Part model, mm, in its own coordinate system. Round coordinates to 2 decimals unless told otherwise and drop trailing zeros. Loops run counter-clockwise (first coordinate to the right, second up) from the corner with the lowest first, then second, coordinate; pieces in that order, holes last.
(1) Cut at B-B on z = 3. List the corners of the cut face in (x, y) (3 decimals), then the cut area to 3 significant figures.
(2) Cut at A-A on y = 60. List the corners of the cut face in (x, z) (3 decimals), then the cut area to 3 significant figures.
(3) Cut at C-C on x = 52. List the corners of the cut face in (y, z), then the cut area to 3 significant figures.
(4) Probe probe 1 along Z at (x, y) = (52, 53); probe 2 along X at (y, z) = (24, 2.4); probe 3 along X at (y, z) = (142, 4.1). List the from-to ranges inside material, lowest first.
from build123d import *

# Parameters (mm, degrees)
F0_W     = 94
F0_H     = 165.2
F1_DEPTH = 6
F2_R     = 2.5
F3_DEPTH = 165.201
F4_SIZE  = 2


with BuildPart() as f1:
    # F0 (on Top) → F1 (new body)
    with BuildSketch(Plane.XY):
        with Locations((47, 82.6)):
            Rectangle(F0_W, F0_H)
    extrude(amount=F1_DEPTH)

    # F2 (on face) → F3 (cut, through all)
    with BuildSketch(Plane.XZ):
        with Locations((42.305, 3)):
            Circle(F2_R)
        with Locations((51.695, 3)):
            Circle(F2_R)
    extrude(amount=-F3_DEPTH, mode=Mode.SUBTRACT)

    # F4
    f4_edges = [f1.edges().sort_by_distance(p)[0] for p in [
        (0, 82.6, 6),
        (0, 82.6, 0),
        (94, 82.6, 6),
        (94, 82.6, 0),
    ]]
    chamfer(f4_edges, length=F4_SIZE)


solid = f1.part
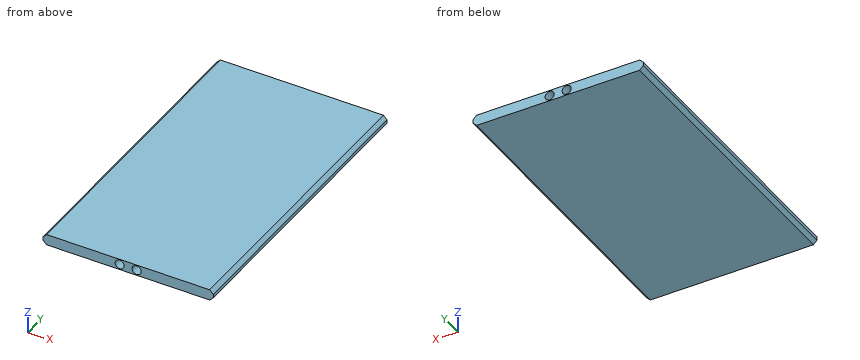
Final values:
1. outline: (0, 0) - (39.805, 0) - (39.805, 165.2) - (0, 165.2) - close; (44.805, 0) - (49.195, 0) - (49.195, 165.2) - (44.805, 165.2) - close; (54.195, 0) - (94, 0) - (94, 165.2) - (54.195, 165.2) - close
1. area: 13,900 mm2
2. outline: (0, 2) - (2, 0) - (92, 0) - (94, 2) - (94, 4) - (92, 6) - (2, 6) - (0, 4) - close; hole circle Ø5 at (42.305, 3); hole circle Ø5 at (51.695, 3)
2. area: 517 mm2
3. outline: (0, 0) - (165.2, 0) - (165.2, 0.52) - (0, 0.52) - close; (0, 5.48) - (165.2, 5.48) - (165.2, 6) - (0, 6) - close
3. area: 171 mm2
4. probe 1: z = 0 to 0.52, 5.48 to 6
4. probe 2: x = 0 to 39.88, 44.73 to 49.27, 54.12 to 94
4. probe 3: x = 0.1 to 40.06, 44.55 to 49.45, 53.94 to 93.9
